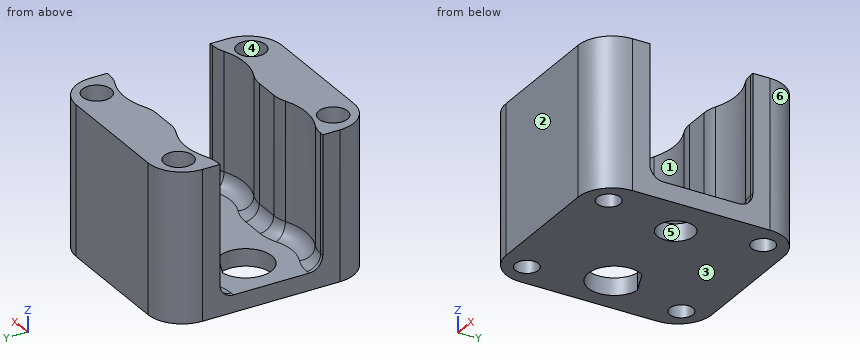
from build123d import *

# Parameters (mm, degrees)
SKETCH1_W               = 34.925
SKETCH1_H               = 38.1
BOSS_EXTRUDE1_DEPTH     = 3.175
SKETCH2_W               = 34.925
SKETCH2_H               = 9.525
BOSS_EXTRUDE2_DEPTH     = 24.3713
CUT_EXTRUDE1_START      = -16.4338
SKETCH3_R               = 11.1125
CUT_EXTRUDE1_DEPTH      = 25.3713
FILLET1_R               = 6.35
FILLET2_R               = 2.54
CUT_EXTRUDE2_DEPTH      = 4.175
F_1_4_CLEARANCE_HOLE1_D = 6.7564
F_6_CLEARANCE_HOLE1_D   = 4.3053
HOLE1_AT_2_COUNT        = 2
HOLE1_AT_2_PITCH        = 25.4
HOLE1_AT_3_COUNT        = 2
HOLE1_AT_3_PITCH        = 28.575
HOLE1_AT_4_COUNT        = 2
HOLE1_AT_4_PITCH        = 38.232062788


with BuildPart() as part:
    # Sketch1 → Boss-Extrude1 (new body)
    with BuildSketch(Plane.XY):
        with Locations((-9.525, 0)):
            Rectangle(SKETCH1_W, SKETCH1_H)
    extrude(amount=BOSS_EXTRUDE1_DEPTH)

    # Sketch2 → Boss-Extrude2 (add)
    with BuildSketch(Plane.XY.offset(3.175)):
        with Locations((-9.525, 14.2875)):
            Rectangle(SKETCH2_W, SKETCH2_H)
    boss_extrude2 = extrude(amount=BOSS_EXTRUDE2_DEPTH)

    # Sketch3 → Cut-Extrude1 (cut)
    with BuildSketch(Plane.XY.offset(19.6088).offset(CUT_EXTRUDE1_START)):
        Circle(SKETCH3_R)
        with Locations((-19.05, 0)):
            Circle(SKETCH3_R)
    cut_extrude1 = extrude(amount=CUT_EXTRUDE1_DEPTH, mode=Mode.SUBTRACT)

    # Mirror1: Boss-Extrude2, Cut-Extrude1 across plane
    add(boss_extrude2.mirror(Plane.ZX))
    add(cut_extrude1.mirror(Plane.ZX), mode=Mode.SUBTRACT)

    # Fillet1
    fillet1_edges = [part.edges().sort_by_distance(p)[0] for p in [
        (7.9375, 19.05, 13.77315),
        (-26.9875, 19.05, 13.77315),
        (5.72381265, 9.525, 15.36065),
        (-5.72381265, 9.525, 15.36065),
        (-13.32618735, 9.525, 15.36065),
        (-24.77381265, 9.525, 15.36065),
        (7.9375, -19.05, 13.77315),
        (-26.9875, -19.05, 13.77315),
        (5.72381265, -9.525, 15.36065),
        (-5.72381265, -9.525, 15.36065),
        (-13.32618735, -9.525, 15.36065),
        (-24.77381265, -9.525, 15.36065),
    ]]
    fillet(fillet1_edges, radius=FILLET1_R)

    # Fillet2
    fillet2_edges = [part.edges().sort_by_distance(p)[0] for p in [
        (7.606169458, 9.525, 3.175),
        (5.921014367, 9.670996527, 3.175),
        (0, 11.1125, 3.175),
        (-5.921014367, 9.670996527, 3.175),
        (-13.128985633, 9.670996527, 3.175),
        (-19.05, 11.1125, 3.175),
        (-24.971014367, 9.670996527, 3.175),
        (-26.656169458, 9.525, 3.175),
        (-9.525, 9.525, 3.175),
        (7.606169458, -9.525, 3.175),
        (5.921014367, -9.670996527, 3.175),
        (0, -11.1125, 3.175),
        (-5.921014367, -9.670996527, 3.175),
        (-9.525, -9.525, 3.175),
        (-13.128985633, -9.670996527, 3.175),
        (-19.05, -11.1125, 3.175),
        (-24.971014367, -9.670996527, 3.175),
        (-26.656169458, -9.525, 3.175),
    ]]
    fillet(fillet2_edges, radius=FILLET2_R)

    # Sketch4 → Cut-Extrude2 (cut, through all)
    with BuildSketch(Plane.XY.offset(3.175)):
        with BuildLine():
            Line((-19.899380011, 4.750666227), (-15.090170105, 2.758627051))
            ThreePointArc((-15.090170105, 2.758627051), (-15.28988845, -3.025200346), (-20.896829618, -4.458642883))
            ThreePointArc((-20.896829618, -4.458642883), (-23.8479402, 0.519659348), (-19.899380011, 4.750666227))
        make_face()
    extrude(amount=-CUT_EXTRUDE2_DEPTH, mode=Mode.SUBTRACT)

    # 1/4 Clearance Hole1 (through all)
    with Locations(Plane.XY.offset(3.175)):
        with Locations((0, 0)):
            Hole(F_1_4_CLEARANCE_HOLE1_D / 2)

    # #6 Clearance Hole1 (through all)
    with Locations(Plane(origin=(0, 0, 0), x_dir=(-1, 0, 0), z_dir=(0, 0, -1))):
        with Locations((-3.175, 14.2875), (22.225, 14.2875), (22.225, -14.2875), (-3.175, -14.2875)):
            Hole(F_6_CLEARANCE_HOLE1_D / 2)

    # Sketch9 → Hole1 (revolve, cut)
    with BuildSketch(Plane(origin=(-22.225, 14.2875, 27.5463), x_dir=(0, -1, 0), z_dir=(1, 0, 0))):
        Polygon((0, 0), (0, 3.81), (2.5273, 3.81), (2.6543, 0), align=None)
    hole1 = revolve(axis=Axis((-22.225, 14.2875, -82.4537), (0, 0, 1)), mode=Mode.SUBTRACT)

    # Hole1 at 2: Hole1 ×2
    with Locations(*[(i * HOLE1_AT_2_PITCH, 0, 0) for i in range(1, HOLE1_AT_2_COUNT)]):
        add(hole1, mode=Mode.SUBTRACT)

    # Hole1 at 3: Hole1 ×2
    with Locations(*[(0, -i * HOLE1_AT_3_PITCH, 0) for i in range(1, HOLE1_AT_3_COUNT)]):
        add(hole1, mode=Mode.SUBTRACT)

    # Hole1 at 4: Hole1 ×2
    with Locations(*[Vector(0.664363839, -0.747409319, 0) * (i * HOLE1_AT_4_PITCH) for i in range(1, HOLE1_AT_4_COUNT)]):
        add(hole1, mode=Mode.SUBTRACT)


solid = part.part
Work out the finished part from the listing and answer in its coordinate system (mm). Face numbers are marked on the shaded views. A direction names the side the tool comes from. Give positions to 0.01 mm unless a question says otherwise; leave off trailing zeros. Write each loop counter-clockwise with the first axis right and the second up, starting at its lowest first coordinate (ties: lowest second). Pieces come first, ordered by that corner, then holes.
Q1. Straight lines are drawn through the part: L1, parallel to Y at x = 0, z = 0.85; L2, parallel to Y at x = -10.5, z = 14.5 (3 decimals); L3, parallel to X at y = -2, z = 2. For each, find the intervals that lie inside material, in ascending order.
Answer:
L1: y = -19.05 to -3.38, 3.38 to 19.05
L2: y = -19.05 to -9.525, 9.525 to 19.05
L3: x = -26.99 to -23.44, -14.66 to -2.72, 2.72 to 7.94
Q2. Given pin 1 (3.5 mm diameter, centred on x = -22.22, y = 14.29, fed in from +Z); pin 2 (8.5 mm diameter, centred on x = -2.5, y = -1.5, fed in from +Z) (3 decimals); pin 3 (1.5 mm diameter, centred on x = 3, z = 18.5, fed in from -Y); pin 4 (1.5 mm diameter, centred on x = -23.5, z = 16.5, fed in from -Y), each flat-ended and moving along its own axis, determine where each tip first touches the part or whether it passes through.
Answer:
pin 1: passes through
pin 2: stops at z = 3.175
pin 3: stops at y = -19.02
pin 4: stops at y = -18.69
Q3. A tool of negligible diameter and unlimited length cuts with its end or side. For the marked faces 1 and 2, from which of +Z, -Z, +X, -X, +Y, -Y can it reach the whole face along a straight path? Write none if from no direction.
Answer:
face 1: +Z
face 2: +Z, -Z, +X, -X, -Y
Q4. For a pull along X with two mould halves and no side action, classify the marked faces 3, 4, 5 and 6 as released by +X, released by -X, zero draft, split by the parting line, or undercut.
Answer:
face 3: zero draft
face 4: undercut
face 5: undercut
face 6: released by +X
Q5. The part is cut by section C-C on y = 0. Give the vertices of the cut face in (x, z) (1 decimal).
Answer:
outline: (-27, 0) - (-23.9, 0) - (-23.9, 3.2) - (-27, 3.2) - close; (-14.2, 0) - (-3.4, 0) - (-3.4, 3.2) - (-14.2, 3.2) - close; (3.4, 0) - (7.9, 0) - (7.9, 3.2) - (3.4, 3.2) - close
Q6. The part is cut by section B-B on z = 17.5. State how many separate pieces and enclosed holes the cut face has, and give its area (3 significant figures).
Answer:
separate pieces: 2
enclosed holes: 4
area: 522 mm2
